Could you check a few things on this model? Use its own coordinates, in mm. Coordinates: 2 decimals unless noted, no trailing zeros. Order: outer loops, then holes, each group sorted by start corner. A loop starts at its lowest first (then second) coordinate and runs counter-clockwise, first axis right, second up. Notation, with made-up numbers: (31, -8.5) - (63, -8.5) arc R21 ccw to (63, 5.5) - close; hole circle Ø7 at (50, 4.25). An arc over 180 degrees is marked (long way). One line per item, written item: value.
from build123d import *

# Parameters (mm, degrees)
F0_W        = 10
F0_H        = 5
F1_DEPTH    = 1
F2_T1_DEPTH = 15.2867319519
F4_DEPTH    = 25
F6_DEPTH    = 5
F8_DEPTH    = 5
F9_R        = 0.72
F10_DEPTH   = 1


# Not quite as in the source:
# - a fillet or chamfer that OpenCascade refuses, or shapes differently, is made with other operations: its cross-section is extruded or revolved along the edge and cut away or added


with BuildPart() as f1:
    # F0 (on Top) → F1 (new body)
    with BuildSketch(Plane.XY):
        with Locations((5, 2.5)):
            Rectangle(F0_W, F0_H)
    extrude(amount=F1_DEPTH)

    # F2: chamfer of 2 on 2 edges, made by hand

    # F2_s2 → F2_t1 (cut)
    with BuildSketch(Plane.XZ.offset(-10.1433659759)):
        Polygon((0, -1), (2, 1), (0, 1), align=None)
        Polygon((10, -1), (8, 1), (10, 1), align=None)
    extrude(amount=F2_T1_DEPTH, mode=Mode.SUBTRACT)

    # F3 (on face) → F4 (cut)
    with BuildSketch(Plane.XZ):
        with BuildLine():
            Line((5, 0.5), (5, 1))
            Line((5, 1), (2, 1))
            ThreePointArc((2, 1), (3.4793093674, 0.6258562046), (5, 0.5))
        make_face()
        with BuildLine():
            Line((8, 1), (5, 1))
            Line((5, 1), (5, 0.5))
            ThreePointArc((5, 0.5), (6.5206906326, 0.6258562046), (8, 1))
        make_face()
        with BuildLine():
            Line((1.1414213562, 0), (8.8585786438, 0))
            Line((8.8585786438, 0), (7.9732451927, 0.8853334511))
            ThreePointArc((7.9732451927, 0.8853334511), (5, 0.4), (2.0267548073, 0.8853334511))
            Line((2.0267548073, 0.8853334511), (1.1414213562, 0))
        make_face()
    extrude(amount=-F4_DEPTH, mode=Mode.SUBTRACT)

    # F5 (on face) → F6 (join)
    with BuildSketch(Plane.XZ):
        Polygon((8.8956828495, 0.1043171505), (9, 0), (9.3658352271, 0), (9.3658352271, 0.1043171505), align=None)
        Polygon((0.6632895378, 0), (1, 0), (1.1006881325, 0.1006881325), (0.6614453159, 0.0918707301), align=None)
    extrude(amount=-F6_DEPTH)

    # F7 (on face) → F8 (join)
    with BuildSketch(Plane.XZ):
        with BuildLine():
            Line((4.275, 0.4), (5, 0.4))
            ThreePointArc((5, 0.4), (4.6372268408, 0.4070403172), (4.275, 0.4281506663))
            Line((4.275, 0.4281506663), (4.275, 0.4))
        make_face()
        with BuildLine():
            ThreePointArc((5.725, 0.4281506663), (5.3627731592, 0.4070403172), (5, 0.4))
            Line((5, 0.4), (5.725, 0.4))
            Line((5.725, 0.4), (5.725, 0.4281506663))
        make_face()
    extrude(amount=-F8_DEPTH)

    # F9 (on face) → F10 (cut)
    with BuildSketch(Plane(origin=(0, 0, 0.4), x_dir=(1, 0, 0), z_dir=(0, 0, -1))):
        with Locations((5, -2.5)):
            Circle(F9_R)
    extrude(amount=-F10_DEPTH, mode=Mode.SUBTRACT)


solid = f1.part
Item 1: I want a section at B-B on y = 0.45. Please give me the cut outline in (x, z) (3 decimals).
Conclusion:
outline: (0.661, 0.092) - (0.663, 0) - (1.141, 0) - (2.027, 0.885) arc R9.35 ccw to (4.275, 0.428) - (4.275, 0.4) - (5.725, 0.4) - (5.725, 0.428) arc R9.35 ccw to (7.973, 0.885) - (8.859, 0) - (9.366, 0) - (9.366, 0.104) - (8.896, 0.104) - (8, 1) arc R9.25 cw to (2, 1) - (1.101, 0.101) - close
Item 2: I want a section at C-C on x = 4.75. Please give me the cut outline in (y, z), then the cut area to 3 significant figures.
Conclusion:
outline: (0, 0.4) - (1.82, 0.4) - (1.82, 0.5) - (0, 0.5) - close; (3.18, 0.4) - (5, 0.4) - (5, 0.5) - (3.18, 0.5) - close
area: 0.377 mm²
Item 3: I'm going to push a flat-ended pin straight in: pin 1 Ø1.2 at (x, y) = (4.5, 3.5) entering from -Z. Where does the tip first touch, or does it pass through?
Conclusion:
pin 1: z = 0.4
Item 4: I want a section at D-D on x = 3.75. Please give me the cut outline in (y, z).
Conclusion:
outline: (0, 0.48) - (5, 0.48) - (5, 0.58) - (0, 0.58) - close
Item 5: I want a section at A-A on y = 2.5. Please give me the cut outline in (x, z) (3 decimals), then the cut area to 3 significant figures.
Conclusion:
outline: (0.661, 0.092) - (0.663, 0) - (1.141, 0) - (2.027, 0.885) arc R9.35 ccw to (4.275, 0.428) - (4.275, 0.4) - (4.28, 0.4) - (4.28, 0.528) arc R9.25 cw to (2, 1) - (1.101, 0.101) - close; (5.72, 0.4) - (5.725, 0.4) - (5.725, 0.428) arc R9.35 ccw to (7.973, 0.885) - (8.859, 0) - (9.366, 0) - (9.366, 0.104) - (8.896, 0.104) - (8, 1) arc R9.25 cw to (5.72, 0.528) - close
area: 0.812 mm²
Item 6: If I drill on probe 1 along Y at (x, z) = (5, 0.45), over which ranges is the centre line in solid material (lowest first)?
Conclusion:
probe 1: 0 to 1.78, 3.22 to 5
